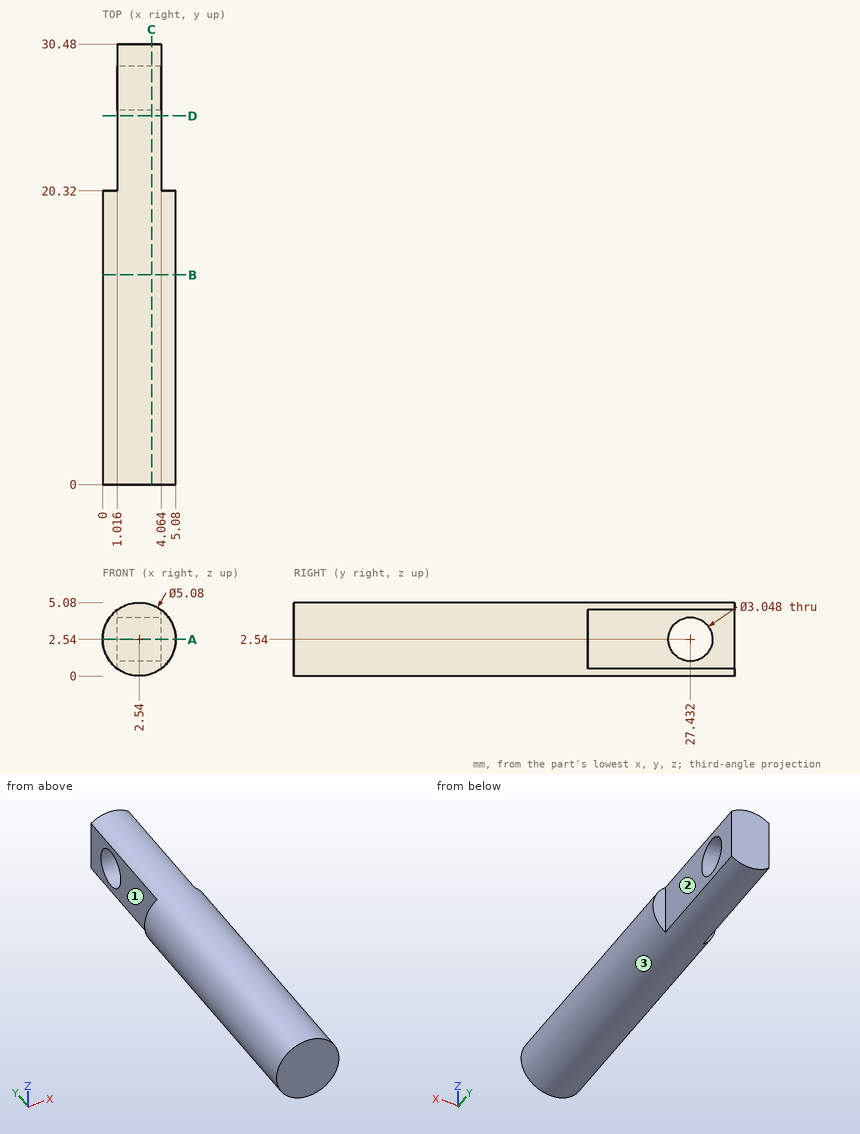
Could you check a few things on this drawing? It's one solid part, dimensions in mm from its lowest x, y, z. A direction names the side the tool comes from. Give positions to 0.01 mm unless a question says otherwise; leave off trailing zeros. Order: outer loops, then holes, each group sorted by start corner. A loop starts at its lowest first (then second) coordinate and runs counter-clockwise, first axis right, second up. Notation, with made-up numbers: (-19, -27) -> (26, -27) arc R25 cw to (26, 9) -> close; hole circle Ø3 at (-36.5, -36.5). An arc over 180 degrees is marked (long way). Use CSV: the item, a comma, the result in double quotes. Start each with the question number.
Item 1: If I drill on probe 1 along Y at (x, z) = (3.15, 2.54); probe 2 along X at (y, z) = (21, 3.15); probe 3 along Y at (x, z) = (4.7, 2.8), over which ranges is the centre line in solid material (lowest first)? Write a range as [from, to].
Item 2: Suppose I cut it at A-A (z = 2.54). List the corners of the cut face in (x, y) for me.
Item 3: On a 3-axis mill with a long thin cutter (end or side, diameter ignored), from which of +Z, -Z, +X, -X, +Y, -Y can I reach the whole of each face in a straight line? I mean the marked faces 1, 2 and 3. Say none if no direction works.
Item 4: I'm going to push flat-ended pins straight in: P1, Ø3, axis at x = 4, y = 4, coming from the +Z side; P2, Ø0.8, axis at x = 4.5, z = 2.5, coming from the +Y side; P3, Ø2, axis at y = 26.5, z = 2.5, coming from the -X side. Where does each tip first touch, or does it pass through?
Item 5: Suppose I cut it at C-C (x = 3.4). List the corners of the cut face in (y, z) for me.
Item 6: Suppose I cut it at B-B (y = 14.5). List the corners of the cut face in (x, z) for me.
Item 7: Suppose I cut it at D-D (y = 25.5). List the corners of the cut face in (x, z) for me, and give its area (3 significant figures).
Answer block:
1,probe 1,"y = [0, 25.91], [28.96, 30.48]"
1,probe 2,"x = [1.02, 4.06]"
1,probe 3,"y = [0, 20.32]"
2,outline,"(0, 0) -> (5.08, 0) -> (5.08, 20.32) -> (4.06, 20.32) -> (4.06, 25.91) -> (1.02, 25.91) -> (1.02, 20.32) -> (0, 20.32) -> close; (1.02, 28.96) -> (4.06, 28.96) -> (4.06, 30.48) -> (1.02, 30.48) -> close"
3,face 1,"+Z, -Z, -X, +Y"
3,face 2,"+Z, -Z, +X, +Y"
3,face 3,"+Y, -Y"
4,P1,"stops at z = 5.08"
4,P2,"stops at y = 20.32"
4,P3,"stops at x = 1.02"
5,outline,"(0, 0.15) -> (30.48, 0.15) -> (30.48, 4.93) -> (0, 4.93) -> close; hole circle Ø3.05 at (27.43, 2.54)"
6,outline,"circle Ø5.08 at (2.54, 2.54)"
7,outline,"(1.02, 0.51) arc R2.54 ccw to (4.06, 0.51) -> (4.06, 4.57) arc R2.54 ccw to (1.02, 4.57) -> close"
7,area,"14.5 mm^2"
